Design review of the part built by this model. Coordinates are the model's own, in mm. A direction names the side the tool comes from. Round coordinates to 2 decimals unless told otherwise and drop trailing zeros. Loops run counter-clockwise (first coordinate to the right, second up) from the corner with the lowest first, then second, coordinate; pieces in that order, holes last. Notation, with made-up numbers: (60, -5.5) -> (119, -5.5) arc R25 cw to (119, 27.5) -> close; hole circle Ø7 at (2.25, -10.75). An arc over 180 degrees is marked (long way). Answer as CSV lines item,"result". Start each with the question number.
```python
from build123d import *

# Parameters (mm, degrees)
ESQUISSE1_W                       = 22
ESQUISSE1_H                       = 230
EXTRUSION1_DEPTH                  = 1.5
DIAM_TRE_DU_PER_AGE_6_0_6_1_D     = 6
DIAM_TRE_DU_PER_AGE_6_0_6_1_DEPTH = 3
DIAM_TRE_DU_PER_AGE_6_0_6_1_TIP   = 1.802581857
ENL_V_MAT_EXTRU_1_REACH           = 5
ENL_V_MAT_EXTRU_2_REACH           = 5
ENL_V_MAT_EXTRU_3_REACH           = 5
ESQUISSE10_R                      = 2.5
EXTRUSION2_DEPTH                  = 3


with BuildPart() as part:
    # Esquisse1 → Extrusion1 (new body, symmetric)
    with BuildSketch(Plane.XY):
        Rectangle(ESQUISSE1_W, ESQUISSE1_H)
    extrude(amount=EXTRUSION1_DEPTH, both=True)

    # Diamètre du perçage Ø6.0 (6)1
    with Locations(Plane.XY.offset(1.5)):
        with Locations((0, 104), (0, -71), (0, -104)):
            Hole(DIAM_TRE_DU_PER_AGE_6_0_6_1_D / 2, depth=DIAM_TRE_DU_PER_AGE_6_0_6_1_DEPTH)
            with Locations((0, 0, -(DIAM_TRE_DU_PER_AGE_6_0_6_1_DEPTH + DIAM_TRE_DU_PER_AGE_6_0_6_1_TIP / 2))):  # 118° drill point
                Cone(0, DIAM_TRE_DU_PER_AGE_6_0_6_1_D / 2, DIAM_TRE_DU_PER_AGE_6_0_6_1_TIP, mode=Mode.SUBTRACT)

    # Esquisse7 → Enlèv. mat.-Extru.1 (cut, up to next)
    with BuildSketch(Plane.XY.offset(1.5), mode=Mode.PRIVATE) as enl_v_mat_extru_1_sk1:
        with BuildLine():
            Line((-4.75, 54.5), (4.75, 54.5))
            ThreePointArc((4.75, 54.5), (5.25, 55), (5.75, 54.5))
            Line((5.75, 54.5), (5.75, 32.5))
            ThreePointArc((5.75, 32.5), (5.25, 32), (4.75, 32.5))
            Line((4.75, 32.5), (-4.75, 32.5))
            ThreePointArc((-4.75, 32.5), (-5.25, 32), (-5.75, 32.5))
            Line((-5.75, 32.5), (-5.75, 54.5))
            ThreePointArc((-5.75, 54.5), (-5.25, 55), (-4.75, 54.5))
        make_face()
    enl_v_mat_extru_1_tool1 = extrude(enl_v_mat_extru_1_sk1.sketch, amount=-ENL_V_MAT_EXTRU_1_REACH, mode=Mode.PRIVATE) & part.part
    add(enl_v_mat_extru_1_tool1.solids().sort_by_distance((0, 43.5, 1.5))[0], mode=Mode.SUBTRACT)

    # Esquisse8 → Enlèv. mat.-Extru.2 (cut, up to next)
    with BuildSketch(Plane.XY.offset(1.5), mode=Mode.PRIVATE) as enl_v_mat_extru_2_sk1:
        with BuildLine():
            Line((-5.5, 0), (5.5, 0))
            ThreePointArc((5.5, 0), (6, -0.5), (5.5, -1))
            Line((5.5, -1), (5.5, -5))
            ThreePointArc((5.5, -5), (6, -5.5), (5.5, -6))
            Line((5.5, -6), (-5.5, -6))
            ThreePointArc((-5.5, -6), (-6, -5.5), (-5.5, -5))
            Line((-5.5, -5), (-5.5, -1))
            ThreePointArc((-5.5, -1), (-6, -0.5), (-5.5, 0))
        make_face()
    enl_v_mat_extru_2_tool1 = extrude(enl_v_mat_extru_2_sk1.sketch, amount=-ENL_V_MAT_EXTRU_2_REACH, mode=Mode.PRIVATE) & part.part
    add(enl_v_mat_extru_2_tool1.solids().sort_by_distance((0, -3, 1.5))[0], mode=Mode.SUBTRACT)

    # Esquisse9 → Enlèv. mat.-Extru.3 (cut, up to next)
    with BuildSketch(Plane.XY.offset(1.5), mode=Mode.PRIVATE) as enl_v_mat_extru_3_sk1:
        with BuildLine():
            Line((-2.5, -19), (4.5, -19))
            ThreePointArc((4.5, -19), (5, -18.5), (5.5, -19))
            Line((5.5, -19), (5.5, -52.5))
            ThreePointArc((5.5, -52.5), (5, -53), (4.5, -52.5))
            Line((4.5, -52.5), (-2.5, -52.5))
            ThreePointArc((-2.5, -52.5), (-3, -53), (-3.5, -52.5))
            Line((-3.5, -52.5), (-3.5, -19))
            ThreePointArc((-3.5, -19), (-3, -18.5), (-2.5, -19))
        make_face()
    enl_v_mat_extru_3_tool1 = extrude(enl_v_mat_extru_3_sk1.sketch, amount=-ENL_V_MAT_EXTRU_3_REACH, mode=Mode.PRIVATE) & part.part
    add(enl_v_mat_extru_3_tool1.solids().sort_by_distance((1, -35.75, 1.5))[0], mode=Mode.SUBTRACT)

    # Esquisse10 → Extrusion2 (add)
    with BuildSketch(Plane.XY.offset(1.5)):
        with Locations((0, 75)):
            Circle(ESQUISSE10_R)
        with Locations((0, -61)):
            Circle(ESQUISSE10_R)
    extrude(amount=EXTRUSION2_DEPTH)


solid = part.part
```
Q1. Add section A-A, the plane y = 104. Give the boundary of the cut face in (x, z), and give its area (3 significant figures).
Q2. Add section D-D, the plane y = 20.5. Give the boundary of the cut face in (x, z).
Q3. Add section B-B, the plane z = 0.6. State how many separate pieces and enclosed holes the cut face has, and give its area (3 significant figures).
Q4. Mouldability with a two-part tool opening along Y and no side actions: class faces 1 (the cylindrical face through (0.65, -73.93, -0.02)), 2 (the flat face through (0, 2, -1.5)) as pulls with the +Y half, pulls with the -Y half, needs draft (parallel to the pull), parting line crosses it, or undercut.
Q5. To check wall thickness, follow probe 1 along Z at (x, y) = (-2.25, -90.5); probe 2 along X at (y, z) = (47, -0.85); probe 3 along X at (y, z) = (104, -0.75). State the ranges of each line that lie inside material, in increasing order. Write a range as from..to.
Q6. For pin 1 Ø3 at (x, z) = (-4.5, 3.5) entering from -Y; pin 2 Ø6.5 at (x, y) = (0.5, 9) entering from +Z, all flat-tipped, find the tip position at first contact; note any pin that passes through.
Q7. Machinability: for faces 3 (the cylindrical face through (0.65, 101.07, -0.02)), 4 (the cylindrical face through (-0.54, 72.56, 2.98)), which of the approach directions +Z, -Z, +X, -X, +Y, -Y give a long, thin tool a straight path to every point of the face, cutting with its end or side? Answer none if there is none.
Q8. Add section C-C, the plane y = -61. Give the boundary of the cut face in (x, z), and give its area (3 significant figures).
Worked answers:
1,outline,"(-11, -1.5) -> (-3, -1.5) -> (-3, 1.5) -> (-11, 1.5) -> close; (3, -1.5) -> (11, -1.5) -> (11, 1.5) -> (3, 1.5) -> close"
1,area,"48.0 mm^2"
2,outline,"(-11, -1.5) -> (11, -1.5) -> (11, 1.5) -> (-11, 1.5) -> close"
3,separate pieces,"1"
3,enclosed holes,"6"
3,area,"4,350 mm^2"
4,face 1,"undercut"
4,face 2,"needs draft"
5,probe 1,"z = -1.5..1.5"
5,probe 2,"x = -11..-5.75, 5.75..11"
5,probe 3,"x = -11..-3, 3..11"
6,pin 1,"passes through"
6,pin 2,"stops at z = 1.5"
7,face 3,"+Z, -Z"
7,face 4,"+Z"
8,outline,"(-11, -1.5) -> (11, -1.5) -> (11, 1.5) -> (2.5, 1.5) -> (2.5, 4.5) -> (-2.5, 4.5) -> (-2.5, 1.5) -> (-11, 1.5) -> close"
8,area,"81.0 mm^2"
